Geometry: final body of the model. Coordinates: model frame, mm. A direction names the side the tool comes from. Give positions to 0.01 mm unless a question says otherwise; leave off trailing zeros. Order: outer loops, then holes, each group sorted by start corner. A loop starts at its lowest first (then second) coordinate and runs counter-clockwise, first axis right, second up. Notation, with made-up numbers: (56.25, -18.5) -> (79.25, -18.5) arc R28 cw to (79.25, 19.5) -> close; hole circle Ø5 at (40.5, 63). An arc over 180 degrees is marked (long way). One line per item, written item: value. Start each with the question number.
```python
from build123d import *

# Parameters (mm, degrees)
F0_R      = 2.6
F1_DEPTH  = 10
F2_R      = 14
F3_DEPTH  = 20
F4_R      = 1.5
F5_DEPTH  = 35.001
F6_SIZE2  = 0.99999
F6_SIZE   = 9.99999
F7_W      = 100
F7_H      = 100
F8_DEPTH  = 3
F10_DEPTH = 25
F11_R     = 5


# Not quite as in the source:
# - a fillet or chamfer is up to 0.001 mm smaller than in the source, because OpenCascade refuses the exact size


with BuildPart() as f1:
    # F0 (on Top) → F1 (new body)
    with BuildSketch(Plane.XY):
        with BuildLine():
            ThreePointArc((8.7499999554, -15.155444592), (15.1554445533, -8.7500000223), (17.5, 0))
            ThreePointArc((17.5, 0), (15.15544445, 8.7500002013), (8.7499995974, 15.1554447987))
            ThreePointArc((8.7499995974, 15.1554447987), (-2.067e-07, 17.5), (-8.7499999554, 15.155444592))
            ThreePointArc((-8.7499999554, 15.155444592), (-15.155444558, 8.7500000142), (-17.5, -1.86e-08))
            ThreePointArc((-17.5, -1.86e-08), (-15.1554444739, -8.7500001599), (-8.7499996963, -15.1554447416))
            ThreePointArc((-8.7499996963, -15.1554447416), (1.496e-07, -17.5), (8.7499999554, -15.155444592))
        make_face()
        Circle(F0_R, mode=Mode.SUBTRACT)
        with BuildLine():
            Line((-17.5, -10.1036297108), (-8.7499996963, -15.1554447416))
            ThreePointArc((-8.7499996963, -15.1554447416), (-15.1554444739, -8.7500001599), (-17.5, -1.86e-08))
            Line((-17.5, -1.86e-08), (-17.5, -10.1036297108))
        make_face()
        with BuildLine():
            Line((0, -20.2072594216), (8.7499999554, -15.155444592))
            ThreePointArc((8.7499999554, -15.155444592), (1.496e-07, -17.5), (-8.7499996963, -15.1554447416))
            Line((-8.7499996963, -15.1554447416), (0, -20.2072594216))
        make_face()
        with BuildLine():
            Line((17.5, -10.1036297108), (17.5, 0))
            ThreePointArc((17.5, 0), (15.1554445533, -8.7500000223), (8.7499999554, -15.155444592))
            Line((8.7499999554, -15.155444592), (17.5, -10.1036297108))
        make_face()
        with BuildLine():
            ThreePointArc((8.7499995974, 15.1554447987), (15.15544445, 8.7500002013), (17.5, 0))
            Line((17.5, 0), (17.5, 10.1036297108))
            Line((17.5, 10.1036297108), (8.7499995974, 15.1554447987))
        make_face()
        with BuildLine():
            ThreePointArc((-8.7499999554, 15.155444592), (-2.067e-07, 17.5), (8.7499995974, 15.1554447987))
            Line((8.7499995974, 15.1554447987), (0, 20.2072594216))
            Line((0, 20.2072594216), (-8.7499999554, 15.155444592))
        make_face()
        with BuildLine():
            ThreePointArc((-17.5, -1.86e-08), (-15.155444558, 8.7500000142), (-8.7499999554, 15.155444592))
            Line((-8.7499999554, 15.155444592), (-17.5, 10.1036297108))
            Line((-17.5, 10.1036297108), (-17.5, -1.86e-08))
        make_face()
    extrude(amount=F1_DEPTH)

    # F2 (on face) → F3 (join)
    with BuildSketch(Plane.XY.offset(10)):
        with BuildLine():
            ThreePointArc((8.7500002145, -15.1554444424), (15.1554446281, -8.7499998928), (17.5, 0))
            ThreePointArc((17.5, 0), (15.1554446281, 8.7499998928), (8.7500002145, 15.1554444424))
            ThreePointArc((8.7500002145, 15.1554444424), (1.496e-07, 17.5), (-8.7499999554, 15.155444592))
            ThreePointArc((-8.7499999554, 15.155444592), (-15.155444558, 8.7500000142), (-17.5, -1.86e-08))
            ThreePointArc((-17.5, -1.86e-08), (-15.1554446126, -8.7499999197), (-8.7500001767, -15.1554444642))
            ThreePointArc((-8.7500001767, -15.1554444642), (2.18e-08, -17.5), (8.7500002145, -15.1554444424))
        make_face()
        Circle(F2_R, mode=Mode.SUBTRACT)
    extrude(amount=F3_DEPTH)

    # F4 (on face) → F5 (cut, through all)
    with BuildSketch(Plane(origin=(-17.5, 0, 0), x_dir=(0, -1, 0), z_dir=(-1, 0, 0))):
        with Locations((0, 5)):
            Circle(F4_R)
    extrude(amount=-F5_DEPTH, mode=Mode.SUBTRACT)

    # F6 (size 10 and 1 in the source; OpenCascade refuses exactly that, so slightly less here)
    f6_edges = [f1.edges().sort_by_distance(p)[0] for p in [
        (14, 0, 20),
        (-14, 0, 10),
        (-14, 0, 30),
    ]]
    f6_side = f1.faces().sort_by_distance((-14, 0, 20))[0]
    chamfer(f6_edges, length=F6_SIZE, length2=F6_SIZE2, reference=f6_side)

    # F7 (on Top) → F8 (join)
    with BuildSketch(Plane.XY):
        Rectangle(F7_W, F7_H)
    extrude(amount=-F8_DEPTH)

    # F9 (on face) → F10 (cut)
    with BuildSketch(Plane.XY):
        Polygon((-40, 40), (-40, 10), (-17.5, 10), (-17.5, 10.1036297108), (-10, 14.4337567297), (-10, 40), align=None)
        Polygon((17.5, 10), (40, 10), (40, 40), (10, 40), (10, 14.4337567297), (17.5, 10.1036297108), align=None)
        Polygon((10, -14.4337567297), (10, -40), (40, -40), (40, -10), (17.5, -10), (17.5, -10.1036297108), align=None)
        Polygon((-40, -10), (-40, -40), (-10, -40), (-10, -14.4337567297), (-17.5, -10.1036297108), (-17.5, -10), align=None)
    extrude(amount=-F10_DEPTH, mode=Mode.SUBTRACT)

    # F11
    f11_edges = [f1.edges().sort_by_distance(p)[0] for p in [
        (-40, 40, -1.5),
        (-10, 40, -1.5),
        (-40, 10, -1.5),
        (10, 40, -1.5),
        (40, 40, -1.5),
        (40, 10, -1.5),
        (40, -10, -1.5),
        (10, -40, -1.5),
        (40, -40, -1.5),
        (-10, -40, -1.5),
        (-40, -40, -1.5),
        (-40, -10, -1.5),
        (50, -50, -1.5),
        (-50, -50, -1.5),
        (-50, 50, -1.5),
        (50, 50, -1.5),
    ]]
    fillet(f11_edges, radius=F11_R)


solid = f1.part
```
1. Access query for faces 4 (the cylindrical face through (38, 11, -2)), 5 (the cylindrical face through (-1.916, 1.757, 4.93)), 6 (the flat face through (-1, -50, -1)), 7 (the flat face through (0, -18, 10)). Directions: +Z, -Z, +X, -X, +Y, -Y. A direction counts if a zero-diameter tool reaches every point of the face in a straight line with its end or side. Return the directions, or none.
2. Cut plane D-D, the plane z = 5. Return loops of the section in (x, y).
3. Material intervals for L1, parallel to Y at x = 0, z = 20; L2, parallel to X at y = -12, z = 12; L3, parallel to Z at x = -34, y = 2.5, sorted ascending. Write a range as [from, to].
4. Cut plane A-A, the plane y = 32. Return loops of the section in (x, z).
5. Cut plane B-B, the plane z = 22. Return loops of the section in (x, y), then the cut area to 3 significant figures.
6. Draft query along X for faces 1 (the cylindrical face through (-12, -39, -2)), 2 (the cylindrical face through (-9.92, 1.5, 5.07)), 3 (the cylindrical face through (48, 49, -2)). Return one class per face: pulls with the +X half, pulls with the -X half, needs draft (parallel to the pull), parting line crosses it, or undercut.
7. Pin query (flat end, axial travel): P1, Ø5, axis at y = 0, z = 5, coming from the -X side; P2, Ø3, axis at y = -7, z = 24.5, coming from the -X side; P3, Ø2, axis at y = 2.5, z = 5, coming from the +X side; P4, Ø2.5, axis at y = 0, z = 5, coming from the -X side. Return the tip coordinate at first contact, or that it passes through.
Answers follow:
1. face 4: +Z, -Z
1. face 5: +Z
1. face 6: +Z, -Z, +X, -X, -Y
1. face 7: +Z, -Y
2. outline: (-17.5, -10.1) -> (0, -20.21) -> (17.5, -10.1) -> (17.5, -1.5) -> (2.12, -1.5) arc R2.6 cw to (-2.12, -1.5) -> (-17.5, -1.5) -> close; (-17.5, 1.5) -> (-2.12, 1.5) arc R2.6 cw to (2.12, 1.5) -> (17.5, 1.5) -> (17.5, 10.1) -> (0, 20.21) -> (-17.5, 10.1) -> close
3. L1: y = [-17.5, -14], [14, 17.5]
3. L2: x = [-12.74, -5.5], [5.5, 12.74]
3. L3: z = [-3, 0]
4. outline: (-50, -3) -> (-40, -3) -> (-40, 0) -> (-50, 0) -> close; (-10, -3) -> (10, -3) -> (10, 0) -> (-10, 0) -> close; (40, -3) -> (50, -3) -> (50, 0) -> (40, 0) -> close
5. outline: circle Ø35 at (0, 0); hole circle Ø28.4 at (0, 0)
5. area: 329 mm²
6. face 1: undercut
6. face 2: needs draft
6. face 3: pulls with the +X half
7. P1: stops at x = -17.5
7. P2: stops at x = -16.61
7. P3: stops at x = 17.5
7. P4: passes through
